Build history of the part. All positions in model axes, mm. A direction names the side the tool comes from. Give positions to 0.01 mm unless a question says otherwise; leave off trailing zeros. Write each loop counter-clockwise with the first axis right and the second up, starting at its lowest first coordinate (ties: lowest second). Pieces come first, ordered by that corner, then holes. Notation, with made-up numbers: (56, 52.25) -> (112, 52.25) arc R4 cw to (112, 59.25) -> close; hole circle Ø6 at (70.5, 1.25). An arc over 180 degrees is marked (long way). One line per question, with ' | ' between items. Start each with the question number.
(1) Band-saw the part on B-B, the plane z = -15. Give the cut face in (x, y).
(2) Band-saw the part on C-C, the plane y = -16.5. Give the cut face in (x, z).
(3) Band-saw the part on A-A, the plane x = 0. Give the cut face in (y, z), and give its area (3 significant figures).
(4) Drill centre lines: probe 1 along X at (y, z) = (-10, -17); probe 2 along Z at (x, y) = (0, 26). Where is each one in solid material? Low to high. Write a range as from..to.
(5) Tool access for faces 1 (the flat face through (-27, 0, -15)), 2 (the cylindrical face through (-6.9, 15.57, -2.49)), 3 (the cylindrical face through (1.302, 26.014, -5.085)): list every direction of +Z, -Z, +X, -X, +Y, -Y with a clear straight run to the whole face (end or side of a thin tool).
(6) Band-saw the part on D-D, the plane z = -26.5. Give the cut face in (x, y).
(7) Pin check, flat tips, straight feed: P1, Ø12, axis at x = -2.5, y = 17.5, coming from the -Z side; P2, Ø12, axis at x = 17.5, y = -8.5, coming from the -Z side; P3, Ø18, axis at x = 0, z = -15, coming from the +Y side. Stop position of each tip, or through.
(8) Pull direction Y, two halves, no side cores. Call faces 4 (the flat face through (0, 20, -4)), 5 (the flat face through (0, 0, 0)), 6 (the flat face through (0, -27, -15)): released by +Y, released by -Y, zero draft, split by the parting line, or undercut.
from build123d import *

# Parameters (mm, degrees)
F0_W     = 54
F0_H     = 54
F0_W_2   = 50
F0_H_2   = 50
F1_DEPTH = 2
F2_DEPTH = 30
F3_R     = 10
F4_DEPTH = 2
F6_DEPTH = 2
F7_R     = 1


with BuildPart() as f1:
    # F0 (on Top) → F1 (new body)
    with BuildSketch(Plane.XY):
        Rectangle(F0_W, F0_H)
        Rectangle(F0_W_2, F0_H_2, mode=Mode.SUBTRACT)
        Rectangle(F0_W_2, F0_H_2)
    extrude(amount=-F1_DEPTH)

    # F0 (on Top) → F2 (join)
    with BuildSketch(Plane.XY):
        Rectangle(F0_W, F0_H)
        Rectangle(F0_W_2, F0_H_2, mode=Mode.SUBTRACT)
    extrude(amount=-F2_DEPTH)

    # F3 (on face) → F4 (cut, through all)
    with BuildSketch(Plane(origin=(0, 27, 0), x_dir=(-1, 0, 0), z_dir=(0, 1, 0))):
        with Locations((0, -15)):
            Circle(F3_R)
    extrude(amount=-F4_DEPTH, mode=Mode.SUBTRACT)

    # F5 (on face) → F6 (join)
    with BuildSketch(Plane(origin=(0, 0, -2), x_dir=(1, 0, 0), z_dir=(0, 0, -1))):
        with BuildLine():
            Line((-7.5, -17), (-7.5, -25))
            Line((-7.5, -25), (7.5, -25))
            Line((7.5, -25), (7.5, -17))
            ThreePointArc((7.5, -17), (6.9142135624, -15.5857864376), (5.5, -15))
            Line((5.5, -15), (-5.5, -15))
            ThreePointArc((-5.5, -15), (-6.9142135624, -15.5857864376), (-7.5, -17))
        make_face()
    extrude(amount=F6_DEPTH)

    # F7
    f7_edges = [f1.edges().sort_by_distance(p)[0] for p in [
        (-7.5, 21, -4),
        (-6.914214, 15.585786, -4),
        (0, 15, -4),
        (6.914214, 15.585786, -4),
        (7.5, 21, -4),
    ]]
    fillet(f7_edges, radius=F7_R)


solid = f1.part
Results:
1) outline: (-27, -27) -> (27, -27) -> (27, 27) -> (10, 27) -> (10, 25) -> (25, 25) -> (25, -25) -> (-25, -25) -> (-25, 25) -> (-10, 25) -> (-10, 27) -> (-27, 27) -> close
2) outline: (-27, -30) -> (-25, -30) -> (-25, -2) -> (25, -2) -> (25, -30) -> (27, -30) -> (27, 0) -> (-27, 0) -> close
3) outline: (-27, -30) -> (-25, -30) -> (-25, -2) -> (15, -2) -> (15, -3) arc R1 ccw to (16, -4) -> (25, -4) -> (25, -5) -> (27, -5) -> (27, 0) -> (-27, 0) -> close; (25, -30) -> (27, -30) -> (27, -25) -> (25, -25) -> close | area: 200 mm²
4) probe 1: x = -27..-25, 25..27 | probe 2: z = -30..-25, -5..0
5) face 1: +Z, -Z, -X, +Y, -Y | face 2: -Z | face 3: +Y
6) outline: (-27, -27) -> (27, -27) -> (27, 27) -> (-27, 27) -> close; hole (-25, -25) -> (25, -25) -> (25, 25) -> (-25, 25) -> close
7) P1: stops at z = -4 | P2: stops at z = -2 | P3: stops at y = -25
8) face 4: undercut | face 5: zero draft | face 6: released by -Y
